Read the model definition and answer for the solid it produces. Units are mm, in the model's axes. Face numbers are marked on the shaded views. A direction names the side the tool comes from. Round coordinates to 2 decimals unless told otherwise and drop trailing zeros. Loops run counter-clockwise (first coordinate to the right, second up) from the corner with the lowest first, then second, coordinate; pieces in that order, holes last. Notation, with made-up numbers: (36, 16) - (73, 16) arc R11 cw to (73, 29) - close; hole circle Ø6 at (85, 36). An arc over 180 degrees is marked (long way). Use CSV: the item, a comma, the result in double quotes. Start each with the question number.
1. Find section A-A (z = 0.5). Give the vertices of the cut face in (x, y).
2. Find section C-C (x = 27.5). Give the vertices of the cut face in (y, z), and give its area (3 significant figures).
3. Find section D-D (x = 3.5). Give the vertices of the cut face in (y, z).
4. Find section B-B (y = 5.5). Give the vertices of the cut face in (x, z), and give its area (3 significant figures).
5. A tool of negligible diameter and unlimited length cuts with its end or side. For the marked faces 1 and 2, from which of +Z, -Z, +X, -X, +Y, -Y can it reach the whole face along a straight path? Write none if from no direction.
6. Consider line 1 along X through (y, z) = (-1.25, 0.7); line 2 along X through (y, z) = (3, 2.65); line 3 along X through (y, z) = (-7.5, 1). Determine where each line is inside the solid, lowest interval first.
7. Given pin 1 Ø1 at (x, z) = (-7, 1.5) entering from +Y; pin 2 Ø1.5 at (x, z) = (27, 2) entering from -Y, each flat-ended and moving along its own axis, determine where each tip first touches the part or whether it passes through.
from build123d import *

# Parameters (mm, degrees)
F0_R     = 4.15
F1_DEPTH = 3


with BuildPart() as f1:
    # F0 (on Top) → F1 (new body)
    with BuildSketch(Plane.XY):
        with BuildLine():
            Line((31.969267, -3.992904), (31.969267, 8.007096))
            Line((31.969267, 8.007096), (9.657442, 8.007096))
            Line((9.657442, 8.007096), (9.774258, 2.39539))
            ThreePointArc((9.774258, 2.39539), (1.864099, -5.824019), (-6.329272, 2.113106))
            ThreePointArc((-6.329272, 2.113106), (-6.330089, 2.22779), (-6.329272, 2.342473))
            Line((-6.329272, 2.342473), (-6.329272, 5.007096))
            ThreePointArc((-6.329272, 5.007096), (-7.207952, 7.128417), (-9.329272, 8.007096))
            Line((-9.329272, 8.007096), (-9.754942, 8.007096))
            ThreePointArc((-9.754942, 8.007096), (-11.876262, 7.128417), (-12.754942, 5.007096))
            Line((-12.754942, 5.007096), (-12.754942, -9.754244))
            ThreePointArc((-12.754942, -9.754244), (-11.876262, -11.875564), (-9.754942, -12.754244))
            Line((-9.754942, -12.754244), (11.273001, -12.754244))
            ThreePointArc((11.273001, -12.754244), (13.394322, -11.875564), (14.273001, -9.754244))
            Line((14.273001, -9.754244), (14.273001, -6.992904))
            ThreePointArc((14.273001, -6.992904), (15.151681, -4.871583), (17.273001, -3.992904))
            Line((17.273001, -3.992904), (31.969267, -3.992904))
        make_face()
        with Locations((24.733823, 1.858876)):
            Circle(F0_R, mode=Mode.SUBTRACT)
        with BuildLine():
            ThreePointArc((-6.329272, 2.342473), (-6.330089, 2.22779), (-6.329272, 2.113106))
            Line((-6.329272, 2.113106), (-6.329272, 2.342473))
        make_face()
    extrude(amount=F1_DEPTH)


solid = f1.part
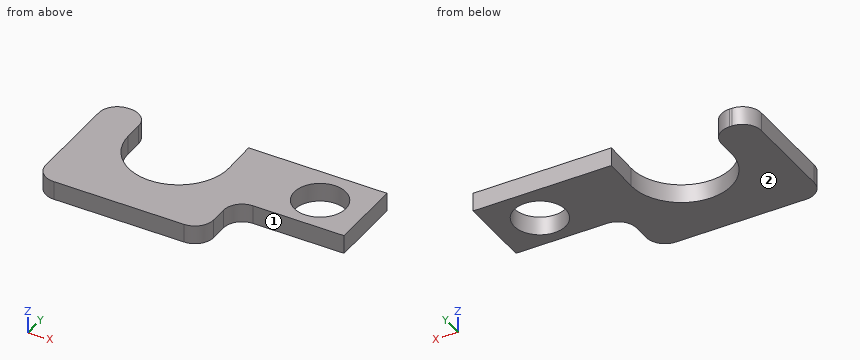
Filled sheet:
1,outline,"(-12.75, -9.75) arc R3 ccw to (-9.75, -12.75) - (11.27, -12.75) arc R3 ccw to (14.27, -9.75) - (14.27, -6.99) arc R3 cw to (17.27, -3.99) - (31.97, -3.99) - (31.97, 8.01) - (9.66, 8.01) - (9.77, 2.4) arc R8.05 cw (long way) to (-6.33, 2.11) - (-6.33, 5.01) arc R3 ccw to (-9.33, 8.01) - (-9.75, 8.01) arc R3 ccw to (-12.75, 5.01) - close; hole circle Ø8.3 at (24.73, 1.86)"
2,outline,"(-3.99, 0) - (-1.23, 0) - (-1.23, 3) - (-3.99, 3) - close; (4.95, 0) - (8.01, 0) - (8.01, 3) - (4.95, 3) - close"
2,area,"17.4 mm²"
3,outline,"(-12.75, 0) - (-5.63, 0) - (-5.63, 3) - (-12.75, 3) - close"
4,outline,"(-12.71, 0) - (-6.37, 0) - (-6.37, 3) - (-12.71, 3) - close; (9.71, 0) - (22.74, 0) - (22.74, 3) - (9.71, 3) - close; (26.72, 0) - (31.97, 0) - (31.97, 3) - (26.72, 3) - close"
4,area,"73.9 mm²"
5,face 1,"+Z, -Z, +X, -Y"
5,face 2,"-Z, +X, -X, +Y, -Y"
6,line 1,"x = -12.75 to -5.54, 8.99 to 21.98, 27.48 to 31.97"
6,line 2,"x = -12.75 to -6.33, 9.76 to 20.74, 28.72 to 31.97"
6,line 3,"x = -12.75 to 14.27"
7,pin 1,"stops at y = 7.38"
7,pin 2,"stops at y = -3.99"
